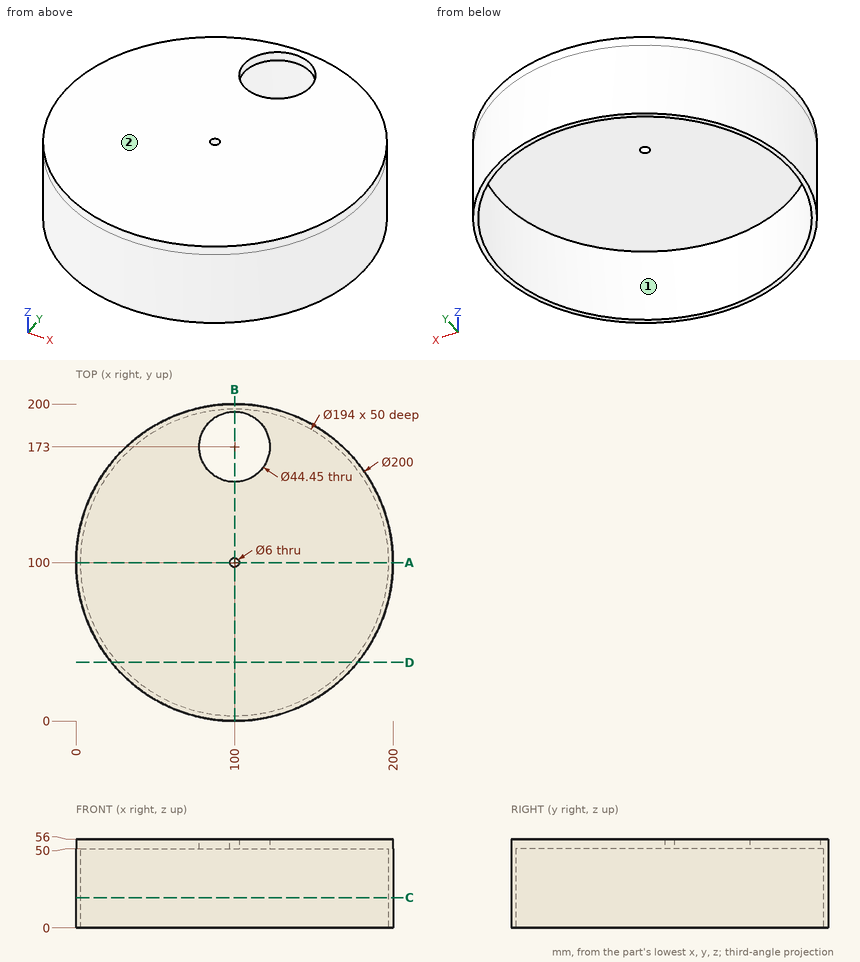
The drawing under review shows one solid part. Ordinate dimensions are in mm from its lowest x, y, z. Round coordinates to 2 decimals unless told otherwise and drop trailing zeros. Write each loop counter-clockwise with the first axis right and the second up, starting at its lowest first coordinate (ties: lowest second). Pieces come first, ordered by that corner, then holes.
(1) We need section B-B on x = 100. Give the boundary of the cut face in (y, z) (3 decimals), and give its area (3 significant figures).
(2) We need section A-A on y = 100. Give the boundary of the cut face in (x, z), and give its area (3 significant figures).
(3) We need section C-C on z = 19. Give the boundary of the cut face in (x, y).
(4) Wall thickness on L1, parallel to Y at x = 100, z = 51.85 (3 decimals); L2, parallel to Y at x = 100, z = 26; L3, parallel to X at y = 102, z = 38.5: over which ranges is each line inside the solid? List them lowest first.
(5) Mouldability with a two-part tool opening along Y and no side actions: class the marked faces 1 and 2 as +Y half, -Y half, draft (parallel to the pull), parting line (faces both ways), or undercut.
(6) Insertion check: pin 1 (3 mm diameter, centred on x = 83.5, z = 35.5, fed in from -Y); pin 2 (1.5 mm diameter, centred on y = 180, z = 29.5, fed in from -X); pin 3 (1 mm diameter, centred on x = 21, z = 20.5, fed in from +Y). Each pin has a flat end and moves straight along its axis. Give the tip position at first contact, or say it passes through.
(7) We need section D-D on y = 37. Give the boundary of the cut face in (x, z).
Findings below:
1. outline: (0, 0) - (3, 0) - (3, 50) - (97, 50) - (97, 56) - (0, 56) - close; (103, 50) - (150.775, 50) - (150.775, 56) - (103, 56) - close; (195.225, 50) - (197, 50) - (197, 0) - (200, 0) - (200, 56) - (195.225, 56) - close
1. area: 1,200 mm2
2. outline: (0, 0) - (3, 0) - (3, 50) - (97, 50) - (97, 56) - (0, 56) - close; (103, 50) - (197, 50) - (197, 0) - (200, 0) - (200, 56) - (103, 56) - close
2. area: 1,460 mm2
3. outline: circle Ø200 at (100, 100); hole circle Ø194 at (100, 100)
4. L1: y = 0 to 97, 103 to 150.775, 195.225 to 200
4. L2: y = 0 to 3, 197 to 200
4. L3: x = 0.02 to 3.02, 196.98 to 199.98
5. face 1: undercut
5. face 2: draft
6. pin 1: stops at y = 1.13
6. pin 2: stops at x = 39.01
6. pin 3: stops at y = 161.95
7. outline: (22.34, 0) - (26.24, 0) - (26.24, 50) - (173.76, 50) - (173.76, 0) - (177.66, 0) - (177.66, 56) - (22.34, 56) - close
